from build123d import *

# Parameters (mm, degrees)
SKETCH1_R                = 68.369999998
SKETCH1_R_2              = 23.401
BOSS_EXTRUDE1_DEPTH      = 2
BOSS_EXTRUDE2_START      = -13
SKETCH3_R                = 68.369999998
SKETCH3_R_2              = 66.37
BOSS_EXTRUDE2_DEPTH      = 13
CUT_EXTRUDE40_DEPTH      = 114.575806629
CUT_EXTRUDE40_DEPTH_BACK = 114.575806629
SKETCH63_R               = 2
CUT_EXTRUDE41_DEPTH      = 160.130961581
CUT_EXTRUDE41_DEPTH_BACK = 160.130961581
SKETCH64_R               = 2
CUT_EXTRUDE45_DEPTH      = 2
SKETCH73_R               = 1
CUT_EXTRUDE47_DEPTH      = 10
SKETCH70_R               = 1.5
CUT_EXTRUDE48_DEPTH      = 10
SKETCH74_R               = 5
CUT_EXTRUDE49_DEPTH      = 10
CUT_EXTRUDE51_START      = -2
CUT_EXTRUDE51_DEPTH      = 2


with BuildPart() as part:
    # Sketch1 → Boss-Extrude1 (new body)
    with BuildSketch(Plane(origin=(0, 0, 0), x_dir=(-0.9985653746512714, 0, -0.053546172109368295), z_dir=(0, 1, 0))):
        with Locations(Location((55.498672647, -32.344920806, 0), (0, 0, 93.069437642))):
            Circle(SKETCH1_R)
        with Locations(Location((55.498672647, -32.344920806, 0), (0, 0, 93.069437642))):
            Circle(SKETCH1_R_2, mode=Mode.SUBTRACT)
    extrude(amount=BOSS_EXTRUDE1_DEPTH)

    # Sketch3 → Boss-Extrude2 (add)
    with BuildSketch(Plane(origin=(0, 2, 0), x_dir=(1, 0, 0), z_dir=(0, 1, 0)).offset(BOSS_EXTRUDE2_START)):
        with Locations(Location((-53.687106148, 35.27025944, 0), (0, 0, 270))):
            Circle(SKETCH3_R)
        with Locations(Location((-53.687106148, 35.27025944, 0), (0, 0, 270))):
            Circle(SKETCH3_R_2, mode=Mode.SUBTRACT)
    extrude(amount=BOSS_EXTRUDE2_DEPTH)

    # Sketch63 → Cut-Extrude40 (cut, two sides: drawn at the far end of the back side and taken through both)
    with BuildSketch(Plane(origin=(-41.506941316, 0, -46.21062949), x_dir=(0.7439552092791144, 2.284460434874975e-13, -0.6682294864688846), z_dir=(0.6682294864688846, -2.5433421830845933e-13, 0.7439552092791144)).offset(-CUT_EXTRUDE40_DEPTH_BACK)):
        with Locations((-16.372174937, -4.35)):
            Circle(SKETCH63_R)
    extrude(amount=CUT_EXTRUDE40_DEPTH + CUT_EXTRUDE40_DEPTH_BACK, mode=Mode.SUBTRACT)

    # Sketch64 → Cut-Extrude41 (cut, two sides: drawn at the far end of the back side and taken through both)
    with BuildSketch(Plane(origin=(-12.180164832, 0, 10.94037005), x_dir=(-0.668229486468876, 1.5883353274739987e-15, -0.743955209279122), z_dir=(0.743955209279122, -1.7683301393964735e-15, -0.668229486468876)).offset(-CUT_EXTRUDE41_DEPTH_BACK)):
        with Locations((62.114800614, -4.35)):
            Circle(SKETCH64_R)
    extrude(amount=CUT_EXTRUDE41_DEPTH + CUT_EXTRUDE41_DEPTH_BACK, mode=Mode.SUBTRACT)

    # Sketch67 → Cut-Extrude45 (cut)
    with BuildSketch(Plane(origin=(0, 2, 0), x_dir=(1, 0, 0), z_dir=(0, 1, 0))):
        with BuildLine():
            Line((-47.831144931, 125.709400378), (-49.82827568, 125.816492726))
            Line((-49.82827568, 125.816492726), (-52.215508738, 81.297751413))
            ThreePointArc((-52.215508738, 81.297751413), (-51.270489538, 80.245639864), (-50.218377989, 81.190659065))
            Line((-50.218377989, 81.190659065), (-47.831144931, 125.709400378))
        make_face()
        with BuildLine():
            Line((-144.126247086, 41.126220657), (-144.233339434, 39.129089908))
            Line((-144.233339434, 39.129089908), (-99.714598121, 36.741856849))
            ThreePointArc((-99.714598121, 36.741856849), (-98.662486572, 37.68687605), (-99.607505773, 38.738987598))
            Line((-99.607505773, 38.738987598), (-144.126247086, 41.126220657))
        make_face()
        with BuildLine():
            Line((36.75203479, 29.414298222), (36.859127139, 31.411428971))
            Line((36.859127139, 31.411428971), (-7.659614175, 33.79866203))
            ThreePointArc((-7.659614175, 33.79866203), (-8.711725723, 32.853642829), (-7.766706523, 31.801531281))
            Line((-7.766706523, 31.801531281), (36.75203479, 29.414298222))
        make_face()
    extrude(amount=-CUT_EXTRUDE45_DEPTH, mode=Mode.SUBTRACT)

    # Sketch73 → Cut-Extrude47 (cut)
    with BuildSketch(Plane.XZ.offset(-2)):
        with Locations(Location((-72.2141021, -18.632644766, 0), (0, 0, 90))):
            Circle(SKETCH73_R)
        with Locations(Location((-37.049491474, -16.743263487, 0), (0, 0, 90))):
            Circle(SKETCH73_R)
        with Locations(Location((-35.160110195, -51.907874114, 0), (0, 0, 90))):
            Circle(SKETCH73_R)
        with Locations(Location((-70.324720822, -53.797255392, 0), (0, 0, 90))):
            Circle(SKETCH73_R)
    extrude(amount=CUT_EXTRUDE47_DEPTH, mode=Mode.SUBTRACT)

    # Sketch70 → Cut-Extrude48 (cut)
    with BuildSketch(Plane(origin=(0, 2, 0), x_dir=(1, 0, 0), z_dir=(0, 1, 0))):
        with Locations(Location((-99.774462502, 65.286181619, 0), (0, 0, 270))):
            Circle(SKETCH70_R)
        with Locations(Location((-56.637979096, -19.650523046, 0), (0, 0, 270))):
            Circle(SKETCH70_R)
        with Locations(Location((-4.648876845, 60.175119746, 0), (0, 0, 270))):
            Circle(SKETCH70_R)
    extrude(amount=-CUT_EXTRUDE48_DEPTH, mode=Mode.SUBTRACT)

    # Sketch74 → Cut-Extrude49 (cut)
    with BuildSketch(Plane(origin=(19.562495047, 3, -2.053609117), x_dir=(1, 0, 0), z_dir=(0, 1, 0))):
        with Locations(Location((-105.702188225, 2.042468777, 0), (0, 0, 270))):
            Circle(SKETCH74_R)
        with Locations(Location((-44.324158759, -1.255349618, 0), (0, 0, 270))):
            Circle(SKETCH74_R)
    extrude(amount=-CUT_EXTRUDE49_DEPTH, mode=Mode.SUBTRACT)

    # Sketch75 → Cut-Extrude51 (cut)
    with BuildSketch(Plane(origin=(0, 2, 0), x_dir=(1, 0, 0), z_dir=(0, 1, 0)).offset(CUT_EXTRUDE51_START)):
        with BuildLine():
            ThreePointArc((-78.28711428, 99.061297209), (-79.21750955, 98.694666428), (-80.142442845, 98.314466628))
            Line((-80.142442845, 98.314466628), (-79.765783898, 97.378744227))
            Line((-79.765783898, 97.378744227), (-71.802851111, 77.596671772))
            ThreePointArc((-71.802851111, 77.596671772), (-70.501771538, 77.04242278), (-69.947522546, 78.343502353))
            Line((-69.947522546, 78.343502353), (-77.910455333, 98.125574808))
            Line((-77.910455333, 98.125574808), (-78.28711428, 99.061297209))
        make_face()
        with BuildLine():
            Line((-21.107609811, 94.229039398), (-20.63291657, 95.119047657))
            ThreePointArc((-20.63291657, 95.119047657), (-21.511818593, 95.596106061), (-22.397604199, 96.060258351))
            Line((-22.397604199, 96.060258351), (-22.872297441, 95.170250092))
            Line((-22.872297441, 95.170250092), (-32.907769586, 76.354618611))
            ThreePointArc((-32.907769586, 76.354618611), (-32.496031118, 75.00166945), (-31.143081956, 75.413407918))
            Line((-31.143081956, 75.413407918), (-21.107609811, 94.229039398))
        make_face()
        with BuildLine():
            Line((-76.23113034, -4.872889039), (-86.266602485, -23.688520519))
            Line((-86.266602485, -23.688520519), (-86.741295726, -24.578528778))
            ThreePointArc((-86.741295726, -24.578528778), (-85.862393702, -25.055587182), (-84.976608096, -25.519739471))
            Line((-84.976608096, -25.519739471), (-84.501914855, -24.629731212))
            Line((-84.501914855, -24.629731212), (-74.46644271, -5.814099732))
            ThreePointArc((-74.46644271, -5.814099732), (-74.878181178, -4.461150571), (-76.23113034, -4.872889039))
        make_face()
        with BuildLine():
            Line((-29.463756963, -27.585055929), (-29.087098016, -28.52077833))
            ThreePointArc((-29.087098016, -28.52077833), (-28.156702745, -28.154147549), (-27.231769451, -27.773947749))
            Line((-27.231769451, -27.773947749), (-27.608428398, -26.838225348))
            Line((-27.608428398, -26.838225348), (-35.571361185, -7.056152893))
            ThreePointArc((-35.571361185, -7.056152893), (-36.872440758, -6.501903901), (-37.42668975, -7.802983474))
            Line((-37.42668975, -7.802983474), (-29.463756963, -27.585055929))
        make_face()
    extrude(amount=CUT_EXTRUDE51_DEPTH, mode=Mode.SUBTRACT)


solid = part.part
Read the model definition and answer for the solid it produces. Units are mm, in the model's axes. A direction names the side the tool comes from. Give positions to 0.01 mm unless a question says otherwise; leave off trailing zeros. Write each loop counter-clockwise with the first axis right and the second up, starting at its lowest first coordinate (ties: lowest second). Pieces come first, ordered by that corner, then holes. Notation, with made-up numbers: M 79,73 L 118,73 A25 cw 118,94 Z; hole C 74,79.5 d10. An arc over 180 degrees is marked long. One line per item, written item: value. Start each with the question number.
(1) Determine the mould class of faces 1 (the cylindrical face through (-33.151, -4.591, 29.943)), 2 (the flat face through (-83, 2, -36)), 3 (the cylindrical face through (-10.175, -4.262, 16.163)) for opening direction X: pulls with the +X half, pulls with the -X half, needs draft (parallel to the pull), parting line crosses it, or undercut.
(2) Find section C-C (y = -9). Determine the outline of the cut face in (x, z), plus the area to 3 significant figures.
(3) Find section A-A (x = -113). Determine the outline of the cut face in (y, z).
(4) A tool of negligible diameter and unlimited length cuts with its end or side. For faces 4 (the flat face through (-53, 0, -7)), 5 (the cylindrical face through (-29.2, 1, 1.5)), from which of +Z, -Z, +X, -X, +Y, -Y can it reach the whole face along a straight path? Write none if from no direction.
(5) Flat-ended cylindrical pins translate along their axes: pin 1 Ø2 at (y, z) = (-5.5, -12) entering from +X; pin 2 Ø1 at (x, y) = (-103.5, -5.5) entering from +Z; pin 3 Ø0.6 at (x, z) = (-50, -103) entering from +Y. Find the tip coordinate at first contact, or state that the pin passes through.
(6) Find section B-B (z = -72). Determine the outline of the cut face in (x, y), plus the area to 3 significant figures.
(7) Find section D-D (x = -60.5). Determine the outline of the cut face in (y, z).
(8) Find the intervals of material crossed by line 1 (Y direction, x = -87, z = -17); line 2 (X direction, y = 1.25, z = -7.5); line 3 (Z direction, x = -11, y = -5), in increasing order.
Results below:
1. face 1: parting line crosses it
1. face 2: needs draft
1. face 3: undercut
2. outline: C -53.69,-35.27 d136.74; hole C -53.69,-35.27 d132.74
2. area: 847 mm^2
3. outline: M -11,-69.28 L 2,-69.28 L 2,-39.46 L 0,-39.46 L 0,-65.05 L -11,-65.05 Z; M -11,-5.49 L 0,-5.49 L 0,-37.45 L 2,-37.45 L 2,-1.26 L -11,-1.26 Z
4. face 4: -Y
4. face 5: +Y, -Y
5. pin 1: stops at x = 10.95
5. pin 2: stops at z = 12.09
5. pin 3: stops at y = 0
6. outline: M -111.35,-11 L -108.97,-11 L -108.97,0 L 1.59,0 L 1.59,-11 L 3.98,-11 L 3.98,2 L -111.35,2 Z
6. area: 283 mm^2
7. outline: M -11,-103.3 L 2,-103.3 L 2,-57.66 L 0,-57.66 L 0,-101.29 L -11,-101.29 Z; M -11,30.75 L 0,30.75 L 0,-12.88 L 2,-12.88 L 2,32.76 L -11,32.76 Z
8. line 1: y = 0 to 2
8. line 2: x = -116.16 to -89.8, -82.48 to 8.79
8. line 3: z = -88.68 to -86.09, 15.55 to 18.14
